Geometry: see drawing. Coordinates: mm, zero at the bounding-box minimum. A direction names the side the tool comes from. Round coordinates to 2 decimals unless told otherwise and drop trailing zeros. Write each loop counter-clockwise with the first axis right and the second up, starting at its lowest first coordinate (ties: lowest second). Pieces come first, ordered by that corner, then holes. Notation, with made-up numbers: M 4,79.5 L 24,79.5 A29 ccw 24,117.5 Z; hole C 15,-29 d8. An arc over 180 degrees is marked long. Write each question's results on one line, items separated by ' | '. Start each with the question number.
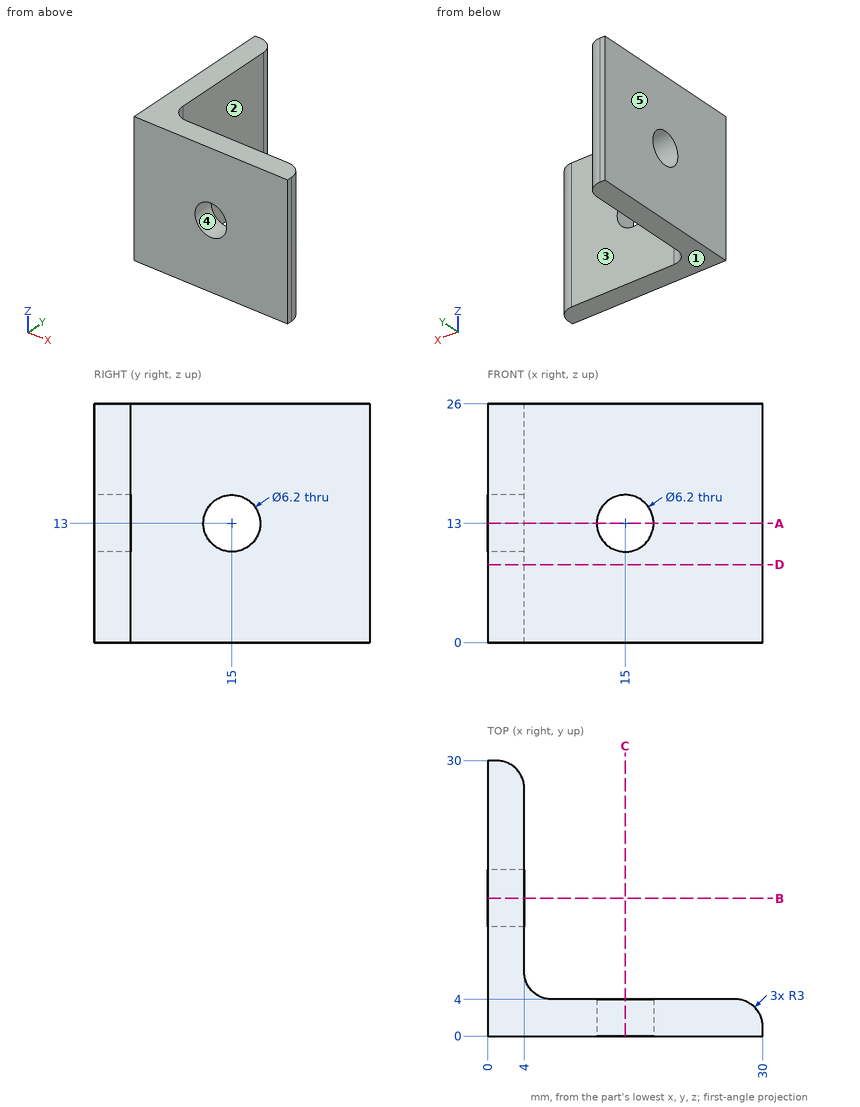
1. Line query: L1, parallel to Z at x = 15, y = 3; L2, parallel to Y at x = 22.5, z = 10.5. Output: solid intervals per line, ascending. Write a range as from..to.
2. Cut plane A-A on z = 13. Output: boundary loops of the cut face in (x, y), and give its area (3 significant figures).
3. Contact query for flat-ended pins moving along their axis: P1, Ø6, axis at x = 14, z = 14, coming from the +Y side; P2, Ø5, axis at x = 15.5, z = 9, coming from the -Y side; P3, Ø1.5, axis at y = 18, z = 13, coming from the +X side. Output: stop coordinate, or through.
4. Draft query along X for the marked faces 3, 4 and 5. Return one class per face: +X half, -X half, draft (parallel to the pull), parting line (faces both ways), or undercut.
5. Cut plane B-B on y = 15. Output: boundary loops of the cut face in (x, z).
6. Access query for the marked faces 1 and 2. Directions: +Z, -Z, +X, -X, +Y, -Y. A direction counts if a zero-diameter tool reaches every point of the face in a straight line with its end or side. Return the directions, or none.
7. Cut plane D-D on z = 8.5. Output: boundary loops of the cut face in (x, y).
Answers follow:
1) L1: z = 0..9.9, 16.1..26 | L2: y = 0..4
2) outline: M 0,0 L 11.9,0 L 11.9,4 L 7,4 A3 cw 4,7 L 4,11.9 L 0,11.9 Z; M 0,18.1 L 4,18.1 L 4,27 A3 ccw 1,30 L 0,30 Z; M 18.1,0 L 30,0 L 30,1 A3 ccw 27,4 L 18.1,4 Z | area: 172 mm2
3) P1: stops at y = 4 | P2: stops at y = 0 | P3: stops at x = 4
4) face 3: draft | face 4: undercut | face 5: -X half
5) outline: M 0,0 L 4,0 L 4,9.9 L 0,9.9 Z; M 0,16.1 L 4,16.1 L 4,26 L 0,26 Z
6) face 1: -Z, +X, -X, +Y, -Y | face 2: +Z, -Z, +X, +Y
7) outline: M 0,0 L 30,0 L 30,1 A3 ccw 27,4 L 7,4 A3 cw 4,7 L 4,27 A3 ccw 1,30 L 0,30 Z
